Model file for the job. Use its own axes, mm. A direction names the side the tool comes from. Give positions to 0.01 mm unless a question says otherwise; leave off trailing zeros. Write each loop counter-clockwise with the first axis right and the second up, starting at its lowest first coordinate (ties: lowest second). Pieces come first, ordered by that corner, then holes. Notation, with made-up numbers: (-0.5, -13) - (36.5, -13) arc R22 ccw to (36.5, 5) - close; hole circle Ø5 at (-38, 61.5). An arc over 180 degrees is marked (long way). Use a Markdown table: item, result. Add a question column.
```python
from build123d import *

# Parameters (mm, degrees)
ESQUISSE1_W             = 105
ESQUISSE1_H             = 75
ESQUISSE1_R             = 2.1
BOSS_EXTRU_1_DEPTH      = 14
ESQUISSE3_W             = 10
ESQUISSE3_H             = 10
ENL_V_MAT_EXTRU_1_DEPTH = 11


with BuildPart() as part:
    # Esquisse1 → Boss.-Extru.1 (new body)
    with BuildSketch(Plane.XY):
        Rectangle(ESQUISSE1_W, ESQUISSE1_H)
        with Locations((47.5, 32.5)):
            Circle(ESQUISSE1_R, mode=Mode.SUBTRACT)
        with Locations(Location((-47.5, 32.5, 0), (0, 0, 180))):
            Circle(ESQUISSE1_R, mode=Mode.SUBTRACT)
        with Locations(Location((47.5, -32.5, 0), (0, 0, 180))):
            Circle(ESQUISSE1_R, mode=Mode.SUBTRACT)
        with Locations((-47.5, -32.5)):
            Circle(ESQUISSE1_R, mode=Mode.SUBTRACT)
    extrude(amount=BOSS_EXTRU_1_DEPTH)

    # Esquisse3 → Enlèv. mat.-Extru.1 (cut)
    with BuildSketch(Plane.XY.offset(14)):
        with Locations((47.5, 32.5)):
            Rectangle(ESQUISSE3_W, ESQUISSE3_H)
        with Locations((-47.5, 32.5)):
            Rectangle(ESQUISSE3_W, ESQUISSE3_H)
        with Locations((-47.5, -32.5)):
            Rectangle(ESQUISSE3_W, ESQUISSE3_H)
        with Locations((47.5, -32.5)):
            Rectangle(ESQUISSE3_W, ESQUISSE3_H)
    extrude(amount=-ENL_V_MAT_EXTRU_1_DEPTH, mode=Mode.SUBTRACT)


solid = part.part
```
(1) Band-saw the part on C-C (z = 10). Write the cut outline in (x, y).
(2) Which spindle directions (+Z, -Z, +X, -X, +Y, -Y) get a long thin tool onto all of the face, cutting with end or side? Do faces 5 (the flat face through (-48, 27.5, 9)), 6 (the cylindrical face through (46.531, -30.637, 1.479)), 7 (the flat face through (42.5, 32, 9)), 8 (the flat face through (47, -27.5, 9)), 9 (the flat face through (-48, -30, 3)). Say none if no direction does.
(3) Probe probe 1 along X at (y, z) = (32.5, 1.05); probe 2 along Y at (x, z) = (47.5, 0.85); probe 3 along X at (y, z) = (-33.5, 4.25). List the from-to ranges inside material, lowest first. Write a range as [from, to].
(4) Band-saw the part on B-B (x = 47.5). Write the cut outline in (y, z), then the cut area to 3 significant figures.
(5) Band-saw the part on A-A (y = 32.5). Write the cut outline in (x, z), then the cut area to 3 significant figures.
(6) Two-plate mould, pull along X, no slides. Class faces 1 (the flat face through (-42.5, -33, 9)), 2 (the flat face through (-1, 1, 0)), 3 (the flat face through (52.5, -1, 7)), 4 (the cylindrical face through (48.469, 30.637, 1.479)): +X half, -X half, draft (parallel to the pull), parting line (faces both ways), or undercut.
(7) Flat gauge pins, fed straight in: pin 1 (5.5 mm diameter, centred on x = -47.5, y = -32.5, fed in from +Z); pin 2 (3 mm diameter, centred on y = 34, z = 10, fed in from +X); pin 3 (8 mm diameter, centred on x = -50, z = 8, fed in from +Y). Where does each tip first touch, or does it go through?
Model answer:
| question | item | result |
|---|---|---|
| 1 | outline | (-52.5, -27.5) - (-42.5, -27.5) - (-42.5, -37.5) - (42.5, -37.5) - (42.5, -27.5) - (52.5, -27.5) - (52.5, 27.5) - (42.5, 27.5) - (42.5, 37.5) - (-42.5, 37.5) - (-42.5, 27.5) - (-52.5, 27.5) - close |
| 2 | face 5 | +Z, -X, +Y |
| 2 | face 6 | +Z, -Z |
| 2 | face 7 | +Z, +X, +Y |
| 2 | face 8 | +Z, +X, -Y |
| 2 | face 9 | +Z, -X, -Y |
| 3 | probe 1 | x = [-52.5, -49.6], [-45.4, 45.4], [49.6, 52.5] |
| 3 | probe 2 | y = [-37.5, -34.6], [-30.4, 30.4], [34.6, 37.5] |
| 3 | probe 3 | x = [-42.5, 42.5] |
| 4 | outline | (-37.5, 0) - (-34.6, 0) - (-34.6, 3) - (-37.5, 3) - close; (-30.4, 0) - (30.4, 0) - (30.4, 3) - (27.5, 3) - (27.5, 14) - (-27.5, 14) - (-27.5, 3) - (-30.4, 3) - close; (34.6, 0) - (37.5, 0) - (37.5, 3) - (34.6, 3) - close |
| 4 | area | 805 mm^2 |
| 5 | outline | (-52.5, 0) - (-49.6, 0) - (-49.6, 3) - (-52.5, 3) - close; (-45.4, 0) - (45.4, 0) - (45.4, 3) - (42.5, 3) - (42.5, 14) - (-42.5, 14) - (-42.5, 3) - (-45.4, 3) - close; (49.6, 0) - (52.5, 0) - (52.5, 3) - (49.6, 3) - close |
| 5 | area | 1,220 mm^2 |
| 6 | face 1 | -X half |
| 6 | face 2 | draft |
| 6 | face 3 | +X half |
| 6 | face 4 | undercut |
| 7 | pin 1 | stops at z = 3 |
| 7 | pin 2 | stops at x = 42.5 |
| 7 | pin 3 | stops at y = 27.5 |
